from build123d import *

# Parameters (mm, degrees)
SKETCH001_R       = 2.355589
SKETCH001_R_2     = 1.789786
SKETCH001_R_3     = 1.472243
SKETCH001_R_4     = 1.183568
SKETCH001_R_5     = 0.92376
PAD_DEPTH         = 15
POCKET_DEPTH      = 8.310486
POCKET_DEPTH_BACK = 1.927638
FILLET_R          = 2
FILLET001_R       = 3.25
CHAMFER_SIZE      = 0.25


with BuildPart() as part:
    # Sketch001 → Pad (new body)
    with BuildSketch(Plane.XY):
        Polygon((0, -8.335405), (24.449893, -6.402758), (24.449893, -1.932647), (0, 0), align=None)
        with Locations((3.855589, -4.167703)):
            Circle(SKETCH001_R, mode=Mode.SUBTRACT)
        with Locations((9.500964, -4.167703)):
            Circle(SKETCH001_R_2, mode=Mode.SUBTRACT)
        with Locations((14.262993, -4.167703)):
            Circle(SKETCH001_R_3, mode=Mode.SUBTRACT)
        with Locations((18.418804, -4.167703)):
            Circle(SKETCH001_R_4, mode=Mode.SUBTRACT)
        with Locations((22.026133, -4.167703)):
            Circle(SKETCH001_R_5, mode=Mode.SUBTRACT)
    extrude(amount=PAD_DEPTH)

    # Sketch002 (on DatumPlane) → Pocket (cut, two sides)
    with BuildSketch(Plane(origin=(0, 0, 0), x_dir=(-0.99689, 0.078799, 0), z_dir=(0.078799, 0.99689, 0))) as pocket_sk:
        Polygon((-26, 15.5), (-26, 7.5), (3, 15.5), align=None)
    extrude(amount=-POCKET_DEPTH, mode=Mode.SUBTRACT)
    extrude(pocket_sk.sketch, amount=POCKET_DEPTH_BACK, mode=Mode.SUBTRACT)

    # Fillet
    fillet_edges = [part.edges().sort_by_distance(p)[0] for p in [
        (24.449893, -6.402758, 3.904703),
        (24.449893, -1.932647, 3.953289),
    ]]
    fillet(fillet_edges, radius=FILLET_R)

    # Fillet001
    fillet001_edges = [part.edges().sort_by_distance(p)[0] for p in [
        (0, -8.335405, 7.24561),
        (0, 0, 7.336207),
    ]]
    fillet(fillet001_edges, radius=FILLET001_R)

    # Chamfer
    chamfer_edges = [part.edges().sort_by_distance(p)[0] for p in [
        (13.056795, -1.032077, 0),
        (13.056795, -1.032077, 11.059304),
        (12.79075, -4.167702, 11.064306),
        (7.711178, -4.167701, 12.46121),
        (17.235236, -4.167702, 9.842054),
        (1.5, -4.167701, 14.169311),
        (21.102372, -4.167702, 8.778575),
        (21.102372, -4.167703, 0),
        (17.235236, -4.167703, 0),
        (12.79075, -4.167703, 0),
        (7.711178, -4.167703, 0),
        (1.5, -4.167703, 0),
    ]]
    chamfer(chamfer_edges, length=CHAMFER_SIZE)


solid = part.part
For this review, take the finished solid that the model builds, in its own axes (mm). Round coordinates to 2 decimals unless told otherwise and drop trailing zeros. Loops run counter-clockwise (first coordinate to the right, second up) from the corner with the lowest first, then second, coordinate; pieces in that order, holes last. Notation, with made-up numbers: (60, 8.25) - (85, 8.25) arc R6 cw to (85, 13.25) - close; hole circle Ø4 at (5.5, 41.25). An arc over 180 degrees is marked (long way). Use one line per item in the form item = value.
Item 1: Consider section B-B on x = 12.25. Write out the cut boundary in (y, z), then the cut area to 3 significant figures.
Answers:
outline = (-7.37, 0.25) - (-7.12, 0) - (-1.22, 0) - (-0.97, 0.25) - (-0.97, 11.02) - (-1.22, 11.28) - (-7.12, 11.15) - (-7.37, 10.88) - close
area = 71.6 mm^2
Item 2: For line 1 (X direction, y = -4, z = 2.5); line 2 (X direction, y = -3.5, z = 1.25); line 3 (Z direction, x = 11.25, y = -2), list the stretches that pass through material, from the lowest coordinate up.
Answers:
line_1 = 0 to 1.51, 6.21 to 7.72, 11.28 to 12.8, 15.73 to 17.25, 19.59 to 21.12, 22.93 to 24.45
line_2 = 0 to 1.6, 6.11 to 7.84, 11.16 to 12.95, 15.58 to 17.44, 19.4 to 21.39, 22.66 to 24.43
line_3 = 0 to 11.54
Item 3: Clearance check with flat-ended pins moving along their axes: P1, Ø1.5, axis at y = -2, z = 6.5, coming from the +X side; P2, Ø2.5, axis at x = 18.42, y = -4.17, coming from the -Z side; P3, Ø1.5, axis at x = 17.5, z = 10, coming from the -Y side. State where each tip first meets the part, or that it passes through.
Answers:
P1 = 24.16
P2 = 0.18
P3 = -7
Item 4: Consider section A-A on z = 4. Write out the cut boundary in (x, y).
Answers:
outline = (0, -4.82) arc R3.25 ccw to (3.51, -8.06) - (22.61, -6.55) arc R2 ccw to (24.45, -4.55) - (24.45, -3.78) arc R2 ccw to (22.61, -1.79) - (3.51, -0.28) arc R3.25 ccw to (0, -3.52) - close; hole circle Ø4.71 at (3.86, -4.17); hole circle Ø3.58 at (9.5, -4.17); hole circle Ø2.94 at (14.26, -4.17); hole circle Ø2.37 at (18.42, -4.17); hole circle Ø1.85 at (22.03, -4.17)
Item 5: Mouldability with a two-part tool opening along Y and no side actions: class faces 1 (the flat face through (12.923, -7.314, 5.224)), 2 (the flat face through (13.191, -1.043, 5.288)), 3 (the flat face through (12, -4, 0)), 4 (the cylindrical face through (12.792, -4.103, 5.46)) as +Y half, -Y half, draft (parallel to the pull), parting line (faces both ways), or undercut.
Answers:
face_1 = -Y half
face_2 = +Y half
face_3 = draft
face_4 = undercut
